from build123d import *

# Parameters (mm, degrees)
F1_R          = 11
F1_R_2        = 4
F2_DEPTH      = 7
F0_R          = 11
F3_DEPTH      = 9
F3_DEPTH_BACK = 2
F4_R          = 2


with BuildPart() as f2:
    # F1 (on Front) → F2 (new body)
    with BuildSketch(Plane.XZ):
        with Locations((0, 24)):
            Circle(F1_R)
        with Locations((0, 24)):
            Circle(F1_R_2, mode=Mode.SUBTRACT)
        with Locations((0, -24)):
            Circle(F1_R)
        with Locations((0, -24)):
            Circle(F1_R_2, mode=Mode.SUBTRACT)
    extrude(amount=F2_DEPTH)


with BuildPart() as f3:
    # F0 (on Front) → F3 (new body, two sides)
    with BuildSketch(Plane.XZ) as f3_sk:
        with BuildLine():
            Line((-8.89, 34.897932), (-8.89, 15.397932))
            ThreePointArc((-8.89, 15.397932), (-17.78, 0), (-8.89, -15.397932))
            Line((-8.89, -15.397932), (-8.89, -34.897932))
            ThreePointArc((-8.89, -34.897932), (0, -37.816214), (8.89, -34.897932))
            Line((8.89, -34.897932), (8.89, -15.397932))
            ThreePointArc((8.89, -15.397932), (17.78, 0), (8.89, 15.397932))
            Line((8.89, 15.397932), (8.89, 34.897932))
            ThreePointArc((8.89, 34.897932), (0, 37.816214), (-8.89, 34.897932))
        make_face()
        Circle(F0_R, mode=Mode.SUBTRACT)
    extrude(amount=F3_DEPTH)
    extrude(f3_sk.sketch, amount=-F3_DEPTH_BACK)

    # F4
    f4_edges = [f3.edges().sort_by_distance(p)[0] for p in [
        (-8.89, -9, 25.147932),
        (-17.78, -9, 0),
        (8.89, -9, 25.147932),
        (17.78, -9, 0),
        (0, -9, 37.816214),
        (0, -9, -37.816214),
        (8.89, -9, -25.147932),
        (-8.89, -9, -25.147932),
        (-8.89, 2, 25.147932),
        (0, 2, 37.816214),
        (-17.78, 2, 0),
        (-8.89, 2, -25.147932),
        (0, 2, -37.816214),
        (8.89, 2, 25.147932),
        (17.78, 2, 0),
        (8.89, 2, -25.147932),
        (-8.89, -3.5, 34.897932),
        (8.89, -3.5, 34.897932),
    ]]
    fillet(f4_edges, radius=F4_R)

    # F5: cut F2
    add(f2.part, mode=Mode.SUBTRACT)


solid = f3.part
Verification items for the finished model (mm, model axes). A direction names the side the tool comes from. Give positions to 0.01 mm unless a question says otherwise; leave off trailing zeros. Loops run counter-clockwise (first coordinate to the right, second up) from the corner with the lowest first, then second, coordinate; pieces in that order, holes last. Notation, with made-up numbers: (-38.75, 79) - (8.25, 79) arc R22 cw to (8.25, 96) - close; hole circle Ø10 at (37.5, -11.75). An arc over 180 degrees is marked (long way). Write item = value, one per line. Start each with the question number.
Q1. Cross-section at C-C, the plane z = -24. Enter the section's corners in (x, y).
Q2. Tool access check on faces 5 (the face through (8.32, -8.4, 24.16)), 6 (the face through (-8.32, -8.4, 23.88)), 7 (the face through (0, -3, 13)), 8 (the face through (8.89, -4, 32)). Record the directions out of +Z, -Z, +X, -X, +Y, -Y that give a thin tool (end or side, any length) a straight path to the whole face; none if there is none.
Q3. Cross-section at B-B, the plane z = 0. Enter the section's corners in (x, y).
Q4. Cross-section at A-A, the plane y = -2.75. Enter the section's corners in (x, z).
Q5. Thickness scan on line 1 (Z direction, x = 0, y = -2); line 2 (Y direction, x = 6, z = -16.5); line 3 (Z direction, x = -6, y = -4.75). Record the ranges inside material, lowest first.
Q6. Mould release check, pull along X, two halves, no side actions. Record for faces 1 (the face through (-0.521, -3.451, 27.966)), 2 (the face through (-4, 0, 27)), 3 (the face through (8.32, 1.4, -24.4)), 4 (the face through (0, -3, 35)): released by +X, released by -X, zero draft, split by the parting line, or undercut.
Q7. Depth check by flat-ended pin: P1, Ø2, axis at x = -2, y = -1, coming from the -Z side; P2, Ø4, axis at y = -5, z = -2, coming from the -X side; P3, Ø0.6, axis at y = -2, z = 16, coming from the +X side; P4, Ø1.5, axis at y = -2, z = 8, coming from the +X side. Enter the tip coordinate at first touch or a pass-through.
Q8. Cross-section at D-D, the plane y = -7.75. Enter the section's corners in (x, z), and give its area (3 significant figures).
Answer key:
q1.outline = (-8.89, -7) arc R2 ccw to (-6.89, -9) - (6.89, -9) arc R2 ccw to (8.89, -7) - (4, -7) - (4, 0) - (8.89, 0) arc R2 ccw to (6.89, 2) - (-6.89, 2) arc R2 ccw to (-8.89, 0) - (-4, 0) - (-4, -7) - close
q2.face_5 = +Z, +X, -Y
q2.face_6 = +Z, -X, -Y
q2.face_7 = none
q2.face_8 = +Z, +X, +Y, -Y
q3.outline = (-17.78, -7) arc R2 ccw to (-15.78, -9) - (-11, -9) - (-11, 2) - (-15.78, 2) arc R2 ccw to (-17.78, 0) - close; (11, -9) - (15.78, -9) arc R2 ccw to (17.78, -7) - (17.78, 0) arc R2 ccw to (15.78, 2) - (11, 2) - close
q4.outline = (-8.89, -34.9) arc R15 ccw to (8.89, -34.9) - (8.89, -30.48) arc R11 cw to (-8.89, -30.48) - close; (-8.89, -17.52) arc R11 cw to (8.89, -17.52) - (8.89, -15.4) arc R17.78 ccw to (8.89, 15.4) - (8.89, 17.52) arc R11 cw to (-8.89, 17.52) - (-8.89, 15.4) arc R17.78 ccw to (-8.89, -15.4) - close; (-8.89, 30.48) arc R11 cw to (8.89, 30.48) - (8.89, 33.84) arc R2 ccw to (7.95, 35.54) arc R15 ccw to (-7.95, 35.54) arc R2 ccw to (-8.89, 33.84) - close; circle Ø8 at (0, -24); circle Ø8 at (0, 24); hole circle Ø22 at (0, 0)
q5.line_1 = -37.82 to -35, -28 to -20, -13 to -11, 11 to 13, 20 to 28, 35 to 37.82
q5.line_2 = -9 to -7, 0 to 2
q5.line_3 = -36.56 to -33.22, -14.78 to -9.22, 9.22 to 14.78, 33.22 to 36.56
q6.face_1 = split by the parting line
q6.face_2 = undercut
q6.face_3 = released by +X
q6.face_4 = undercut
q7.P1 = -37.78
q7.P2 = -17.78
q7.P3 = 8.89
q7.P4 = 16.23
q8.outline = (-8.74, -34.82) arc R14.85 ccw to (8.74, -34.82) - (8.74, -15.31) arc R17.63 ccw to (8.74, 15.31) - (8.74, 33.84) arc R1.85 ccw to (7.87, 35.41) arc R14.85 ccw to (-7.87, 35.41) arc R1.85 ccw to (-8.74, 33.84) - (-8.74, 15.31) arc R17.63 ccw to (-8.74, -15.31) - close; hole circle Ø22 at (0, 0)
q8.area = 1,290 mm^2
